```python
from build123d import *

# Parameters (mm, degrees)
F0_W     = 3
F0_H     = 6
F0_R     = 6.75
F1_DEPTH = 3


with BuildPart() as f1:
    # F0 (on Front) → F1 (new body)
    with BuildSketch(Plane.XZ):
        with BuildLine():
            Line((-46.090017, -19.444276), (-24.535898, -7))
            Line((-24.535898, -7), (18.343146, -7))
            ThreePointArc((18.343146, -7), (21, -8.485281), (24, -9))
            ThreePointArc((24, -9), (27.362164, -8.348404), (30.23749, -6.487968))
            Line((30.23749, -6.487968), (43.227871, -13.987968))
            Line((43.227871, -13.987968), (45.727871, -9.657841))
            Line((45.727871, -9.657841), (32.73749, -2.157841))
            ThreePointArc((32.73749, -2.157841), (31.085921, 5.548848), (24, 9))
            ThreePointArc((24, 9), (21, 8.485281), (18.343146, 7))
            Line((18.343146, 7), (-24, 7))
            ThreePointArc((-24, 7), (-28.141105, 6.454813), (-32, 4.856406))
            Line((-32, 4.856406), (-52.78461, -7.143594))
            ThreePointArc((-52.78461, -7.143594), (-55.069211, -8.743289), (-57.041321, -10.715398))
            Line((-57.041321, -10.715398), (-69.816408, -25.940155))
            ThreePointArc((-69.816408, -25.940155), (-58.754651, -28.314504), (-48.887849, -22.778603))
            Line((-48.887849, -22.778603), (-46.090017, -19.444276))
        make_face()
        with Locations((-24, 0)):
            Rectangle(F0_W, F0_H, mode=Mode.SUBTRACT)
        with Locations((24, 0)):
            Circle(F0_R, mode=Mode.SUBTRACT)
    extrude(amount=F1_DEPTH)


solid = f1.part
```
Geometry check sheet. Reference: the model listing, model coordinates, mm. A direction names the side the tool comes from. Give positions to 0.01 mm unless a question says otherwise; leave off trailing zeros. Order: outer loops, then holes, each group sorted by start corner. A loop starts at its lowest first (then second) coordinate and runs counter-clockwise, first axis right, second up. Notation, with made-up numbers: (37.25, -7) - (51.25, -7) arc R10 cw to (51.25, 8) - close; hole circle Ø6 at (38, -7.5). An arc over 180 degrees is marked (long way). Answer in a Markdown table with one row per item. Add a question column.
Q1. Cross-section at D-D, the plane z = -4.5. Enter the section's corners in (x, y), then the cut area to 3 significant figures.
Q2. Mould release check, pull along X, two halves, no side actions. Record for faces 4 (the flat face through (-22.5, -1, 0)), 5 (the cylindrical face through (-28.08, -1.48, 6.47)), 6 (the flat face through (-3, -1, 7)): pulls with the +X half, pulls with the -X half, needs draft (parallel to the pull), parting line crosses it, or undercut.
Q3. Cross-section at B-B, the plane y = -1. Enter the section's corners in (x, z).
Q4. Tool access check on faces 1 (the flat face through (-24, -1, -3)), 2 (the flat face through (-35.464, -1.479, -13.309)), 3 (the flat face through (44.46, -1.48, -11.85)). Record the directions out of +Z, -Z, +X, -X, +Y, -Y that give a thin tool (end or side, any length) a straight path to the whole face; none if there is none.
Q5. Cross-section at C-C, the plane x = 19.5. Enter the section's corners in (y, z), then the cut area to 3 significant figures.
Q6. Material ranges on probe 1 along X at (y, z) = (-1.3, 1); probe 2 along Z at (x, y) = (-13.5, -2.7); probe 3 along Z at (x, y) = (24.5, -1.6), recorded low to high. Write a range as from..to.
Q7. Gauge pin test, flat ends, axial feed: pin 1 (1.5 mm diameter, centred on x = 5.5, y = -1, fed in from +Z); pin 2 (1 mm diameter, centred on x = -23, y = -0.5, fed in from -Z); pin 3 (1 mm diameter, centred on y = -1, z = -13, fed in from -X). Record the tip position at first contact, or that the pin passes through.
Q8. Cross-section at A-A, the plane z = 0. Enter the section's corners in (x, y).
Check values:
| question | item | result |
|---|---|---|
| 1 | outline | (-48.21, -3) - (18.97, -3) - (18.97, 0) - (-48.21, 0) - close; (29.03, -3) - (36.79, -3) - (36.79, 0) - (29.03, 0) - close |
| 1 | area | 225 mm^2 |
| 2 | face 4 | undercut |
| 2 | face 5 | pulls with the -X half |
| 2 | face 6 | needs draft |
| 3 | outline | (-69.82, -25.94) arc R16 ccw to (-48.89, -22.78) - (-46.09, -19.44) - (-24.54, -7) - (18.34, -7) arc R9 ccw to (24, -9) arc R9 ccw to (30.24, -6.49) - (43.23, -13.99) - (45.73, -9.66) - (32.74, -2.16) arc R9 ccw to (24, 9) arc R9 ccw to (18.34, 7) - (-24, 7) arc R16 ccw to (-32, 4.86) - (-52.78, -7.14) arc R16 ccw to (-57.04, -10.72) - close; hole (-25.5, -3) - (-22.5, -3) - (-22.5, 3) - (-25.5, 3) - close; hole circle Ø13.5 at (24, 0) |
| 4 | face 1 | +Y, -Y |
| 4 | face 2 | -Z, +Y, -Y |
| 4 | face 3 | -Z, +X, +Y, -Y |
| 5 | outline | (-3, -7.79) - (0, -7.79) - (0, -5.03) - (-3, -5.03) - close; (-3, 5.03) - (0, 5.03) - (0, 7.79) - (-3, 7.79) - close |
| 5 | area | 16.6 mm^2 |
| 6 | probe 1 | x = -38.68..-25.5, -22.5..17.32, 30.68..32.94 |
| 6 | probe 2 | z = -7..7 |
| 6 | probe 3 | z = -8.99..-6.73, 6.73..8.99 |
| 7 | pin 1 | stops at z = 7 |
| 7 | pin 2 | stops at z = -7 |
| 7 | pin 3 | stops at x = -59.38 |
| 8 | outline | (-40.41, -3) - (-25.5, -3) - (-25.5, 0) - (-40.41, 0) - close; (-22.5, -3) - (17.25, -3) - (17.25, 0) - (-22.5, 0) - close; (30.75, -3) - (33, -3) - (33, 0) - (30.75, 0) - close |
